Autodesk Inventor part; units mm, degrees
ref_plane "YZ Plane" through (0, 0, 0) normal (1, 0, 0) x (0, 1, 0)
ref_plane "XZ Plane" through (0, 0, 0) normal (0, 1, 0) x (-1, 0, 0)
ref_plane "XY Plane" through (0, 0, 0) normal (0, 0, 1) x (1, 0, 0)
sketch "Sketch1" plane through (0, 0, 0) normal (0, 1, 0) x (-1, 0, 0)
  circle A0 centre (0, 0) radius 57
  circle A1 centre (0, 0) radius 50
  line L0 (0, -85.4) -> (0, 113.4)
  line L1 (112.682, 0) -> (-112.682, 0)
  line L2 (-50, 2) -> (50, 2)
  line L3 (50, 2) -> (50, -2)
  line L4 (50, -2) -> (-50, -2)
  line L5 (-50, -2) -> (-50, 2)
  line L6 (-50, 2) -> (50, -2) construction
  line L7 (50, 2) -> (-50, -2) construction
  line L8 (2, 50) -> (-2, 50)
  line L9 (-2, 50) -> (-2, -50)
  line L10 (-2, -50) -> (2, -50)
  line L11 (2, -50) -> (2, 50)
  line L12 (2, 50) -> (-2, -50) construction
  line L13 (-2, 50) -> (2, -50) construction
  line L14 (13.75, 85) -> (-13.75, 85)
  line L15 (-13.75, 85) -> (-13.75, 50)
  line L16 (-13.75, 50) -> (13.75, 50)
  line L17 (13.75, 50) -> (13.75, 85)
  line L18 (0, 85) -> (0, 50) construction
  line L19 (13.75, 60) -> (-13.75, 60)
  line L20 (-44.3013, -23.2679) -> (-42.3013, -26.7321)
  line L21 (-36.4263, -36.9078) -> (-50.1763, -13.0922)
  line L22 (-58.8365, -18.0922) -> (-45.0865, -41.9078)
  line L23 (-66.7372, -54.4078) -> (-36.4263, -36.9078)
  line L24 (-50.1763, -13.0922) -> (-80.4872, -30.5922)
  line L25 (-73.6122, -42.5) -> (-43.3013, -25) construction
  line L26 (-80.4872, -30.5922) -> (-66.7372, -54.4078)
  line L27 (42.3013, -26.7321) -> (44.3013, -23.2679)
  line L28 (50.1763, -13.0922) -> (36.4263, -36.9078)
  line L29 (45.0865, -41.9078) -> (58.8365, -18.0922)
  line L30 (80.4872, -30.5922) -> (50.1763, -13.0922)
  line L31 (36.4263, -36.9078) -> (66.7372, -54.4078)
  line L32 (73.6122, -42.5) -> (43.3013, -25) construction
  line L33 (66.7372, -54.4078) -> (80.4872, -30.5922)
  point P0 (2, -49.96)
  point P1 (2, -2)
  point P2 (49.96, -2)
  point P3 (-2, 49.96)
  point P4 (-2, 2)
  point P5 (-49.96, 2)
  point P6 (-2, -49.96)
  point P7 (-49.96, -2)
  point P8 (-2, -2)
  point P9 (-13.75, 55.3167)
  point P10 (-54.7807, -15.7505)
  point P11 (-41.0307, -39.5662)
  point P12 (41.0307, -39.5662)
  point P13 (54.7807, -15.7505)
  point P14 (13.75, 55.3167)
  point P15 (2, 49.96)
  point P16 (49.96, 2)
  point P17 (2, 2)
  dimension "d0" = 114
  dimension "d1" = 100
  dimension "d6" = 100
  dimension "d7" = 4
  dimension "d8" = 4
  dimension "d9" = 100
  dimension "d10" = 27.5
  dimension "d14" = 60
  dimension "d15" = 25
  dimension "d18" = 360
extrude "Extrusion1" add sketch "Sketch1" along normal blind 5 contours L1 L3 L2 A1 L11 L16 L17 A0 | A0 L30 L28 L27 A1 L4 L3 L1 | L17 L16 L8 L0 A0 | A0 L0 L19 L17 | L30 L29 L31 A0 | A0 L31 L28 L27 L30 | L1 L11 L2 A1 | L3 L4 A1 | A1 L4 L11 L1 | A1 L2 L3 | L0 L8 L16 L15 A0 | A0 L15 L19 L0 | L19 L0 L14 L17 | A0 L0 L10 L11 A1 L27 L28 L31 | L30 L33 L31 L29 | L11 L4 L0 L1 | L1 L0 L2 L11 | L15 L16 L9 A1 L2 L5 L1 A0 | L8 L11 A1 | L0 L2 L9 A1 | A1 L11 L2 L0 | A1 L9 L8 | L19 L15 L14 L0 | A0 L23 L21 L20 A1 L9 L10 L0 | L11 A1 L0 L4 | L1 L9 L2 L0 | L0 L4 L9 L1 | L1 L5 L4 A1 L20 L21 L24 A0 | L23 L22 L24 A0 | A0 L24 L21 L20 L23 | L10 L9 A1 | A1 L9 L4 L0 | A1 L11 L10 | L9 L4 A1 L1 | L1 A1 L2 L9 | L5 L2 A1 | A1 L4 L5 | L23 L26 L24 L22
sketch "Sketch5" plane through (0, 5, 0) normal (0, 1, 0) x (1, 0, 0)
  line L0 (-2, -21.5) -> (2, -21.5)
  line L1 (2, -21.5) -> (2, -17.5)
  line L2 (2, -17.5) -> (-2, -17.5)
  line L3 (-2, -17.5) -> (-2, -21.5)
  line L4 (-2, -2) -> (-2, -49.96) construction
  line L5 (2, -49.96) -> (2, -2) construction
  line L6 (-112.682, 0) -> (112.682, 0) construction
  line L7 (-2, 21.5) -> (2, 21.5)
  line L8 (2, 21.5) -> (2, 17.5)
  line L9 (2, 17.5) -> (-2, 17.5)
  line L10 (-2, 17.5) -> (-2, 21.5)
  arc A0 (-49.96, -2) -> (-2, -49.96) centre (0, 0) ccw construction
  arc A1 (-2, 49.96) -> (-49.96, 2) centre (0, 0) ccw construction
  circle A2 centre (0, 0) radius 50 construction
  line L11 (-54, 6) -> (-50, 6)
  line L12 (-50, 6) -> (-50, -6)
  line L13 (-50, -6) -> (-54, -6)
  line L14 (-54, -6) -> (-54, 6)
  line L15 (-54, 0) -> (-50, 0) construction
  line L16 (0, 88.2024) -> (0, -113.8671) construction
  line L17 (54, 6) -> (50, 6)
  line L18 (50, 6) -> (50, -6)
  line L19 (50, -6) -> (54, -6)
  line L20 (54, -6) -> (54, 6)
  line L21 (54, 0) -> (50, 0) construction
  point P0 (49.96, -2)
  point P1 (49.96, 2)
  dimension "d41" = 17.5
  dimension "d42" = 4
  dimension "d43" = 12
extrude "Extrusion4" add sketch "Sketch5" along normal blind 10
sketch "Sketch2" plane through (0, 5, 0) normal (0, 1, 0) x (1, 0, 0)
  line L0 (-13.75, -55.3167) -> (-13.75, -85)
  line L1 (13.75, -85) -> (13.75, -55.3167)
  line L2 (-13.75, -85) -> (13.75, -85)
  line L3 (13.75, -85) -> (13.75, -61)
  line L4 (13.75, -61) -> (-13.75, -61)
  line L5 (-13.75, -61) -> (-13.75, -85)
  line L6 (-12.25, -62.5) -> (12.25, -62.5)
  line L7 (12.25, -62.5) -> (12.25, -83.5)
  line L8 (12.25, -83.5) -> (-12.25, -83.5)
  line L9 (-12.25, -83.5) -> (-12.25, -62.5)
  line L10 (80.4872, 30.5922) -> (66.7372, 54.4078)
  line L11 (66.7372, 54.4078) -> (45.9525, 42.4078)
  line L12 (45.9525, 42.4078) -> (59.7025, 18.5922)
  line L13 (59.7025, 18.5922) -> (80.4872, 30.5922)
  line L14 (60.2516, 20.6412) -> (48.0016, 41.8588)
  line L15 (48.0016, 41.8588) -> (66.1881, 52.3588)
  line L16 (66.1881, 52.3588) -> (78.4381, 31.1412)
  line L17 (78.4381, 31.1412) -> (60.2516, 20.6412)
  line L18 (-66.7372, 54.4078) -> (-80.4872, 30.5922)
  line L19 (-80.4872, 30.5922) -> (-59.7025, 18.5922)
  line L20 (-59.7025, 18.5922) -> (-45.9525, 42.4078)
  line L21 (-45.9525, 42.4078) -> (-66.7372, 54.4078)
  line L22 (-48.0016, 41.8588) -> (-60.2516, 20.6412)
  line L23 (-60.2516, 20.6412) -> (-78.4381, 31.1412)
  line L24 (-78.4381, 31.1412) -> (-66.1881, 52.3588)
  line L25 (-66.1881, 52.3588) -> (-48.0016, 41.8588)
  point P0 (0, 0)
  point P1 (-13.75, -61)
  point P2 (-13.75, -61)
  dimension "d22" = 24
  dimension "d23" = 1.5
  dimension "d26" = 360
extrude "Extrusion2" add sketch "Sketch2" along normal blind 20 contours L4 L1 L2 L0
sketch "Sketch4" plane through (-13.75, 0, 85) normal (0, 0, 1) x (1, 0, 0)
  line L0 (0, 25) -> (27.5, 25) construction
  line L1 (7.75, 25) -> (19.75, 25)
  line L2 (19.75, 25) -> (19.75, 10)
  line L3 (19.75, 10) -> (7.75, 10)
  line L4 (7.75, 10) -> (7.75, 25)
  line L5 (1.5, 5) -> (26, 5) construction
  line L6 (13.75, -10.2) -> (13.75, 61.2) construction
  circle A0 centre (13.75, 16) radius 6
  point P0 (13.75, 0)
  point P1 (7.75, 16)
  point P2 (19.75, 16)
  dimension "d36" = 12
  dimension "d37" = 5
  dimension "d38" = 6
extrude "Extrusion3" cut sketch "Sketch4" against normal up to surface (24 mm away) contours L1 L2 A0 L4 | A0
pattern_circular "Circular Pattern1" count 3 over 360 about axis through (0, -10, 0) along (0, 1, 0) of "Extrusion2", "Extrusion3"
equation "\"d38\" = 0.5 * d36"
properties part number "bottom3"
Read the model definition and answer for the solid it produces. Units are mm, in the model's axes. A direction names the side the tool comes from. Round coordinates to 2 decimals unless told otherwise and drop trailing zeros. Loops run counter-clockwise (first coordinate to the right, second up) from the corner with the lowest first, then second, coordinate; pieces in that order, holes last.
Q1. Which of the six approach directions +Z, -Z, +X, -X, +Y, -Y give full straight-line access (tool end or side, diameter ignored) to faces 4 (the face through (2, 4, -26)), 5 (the face through (-52, 10, -6)), 6 (the face through (12.25, 15, 73)), 7 (the face through (50, 10, 0)), 8 (the face through (-52, 10, 6))?
Q2. Determine the mould class of faces 1 (the face through (0, 15, -20)), 2 (the face through (52, 10, 6)), 3 (the face through (49.681, 2.465, 27.943)) for opening direction Z: released by +Z, released by -Z, zero draft, split by the parting line, or undercut.
Q3. Consider probe 1 along Z at (x, y) = (-52, 7); probe 2 along Z at (x, y) = (9, 21.5); probe 3 along Z at (x, y) = (-16, 2). Determine where each line is inside the solid, lowest interval first.
Q4. Each of these flat-tipped pins is pushed along its axis until it touches: pin 1 (0.8 mm diameter, centred on y = 21.5, z = 84.5, fed in from -X); pin 2 (2 mm diameter, centred on x = -52, y = 9, fed in from +Z); pin 3 (2.5 mm diameter, centred on x = 36.5, y = 3.5, fed in from -Z); pin 4 (10 mm diameter, centred on y = 21, z = 16, fed in from -X). Where does it stop, or does it pass through?
Q5. Section B-B on z = 44 is taken. Write down the section's boundary in (x, y), and give its area (3 significant figures).
Q6. Section A-A on y = 3 is taken. Write down the section's boundary in (x, z).
Q7. Section C-C on x = -30 is taken. Write down the section's boundary in (y, z), and give its area (3 significant figures).
Output:
1. face 4: +Y, -Y
1. face 5: +X, -X, +Y
1. face 6: +Y
1. face 7: +Z, +Y
1. face 8: +Z, +X, -X, +Y
2. face 1: zero draft
2. face 2: released by +Z
2. face 3: undercut
3. probe 1: z = -45.9 to -44.17, -34.93 to -31.93, -6 to 6
3. probe 2: z = 61 to 62.5, 83.5 to 85
3. probe 3: z = -54.71 to -47.37, -2 to 2, 47.37 to 54.71
4. pin 1: stops at x = -13.75
4. pin 2: stops at z = 6
4. pin 3: stops at z = -44.79
4. pin 4: passes through
5. outline: (-36.24, 0) - (-23.75, 0) - (-23.75, 5) - (-36.24, 5) - close; (-2, 0) - (2, 0) - (2, 5) - (-2, 5) - close; (23.75, 0) - (36.24, 0) - (36.24, 5) - (23.75, 5) - close
5. area: 145 mm2
6. outline: (-80.49, -30.59) - (-66.74, -54.41) - (-41.03, -39.57) arc R57 ccw to (41.03, -39.57) - (66.74, -54.41) - (80.49, -30.59) - (54.78, -15.75) arc R57 ccw to (13.75, 55.32) - (13.75, 85) - (-13.75, 85) - (-13.75, 55.32) arc R57 ccw to (-54.78, -15.75) - close; hole (-49.96, -2) arc R50 ccw to (-2, -49.96) - (-2, -2) - close; hole (-49.96, 2) - (-2, 2) - (-2, 49.96) arc R50 ccw to start; hole (2, -49.96) arc R50 ccw to (49.96, -2) - (2, -2) - close; hole (2, 2) - (49.96, 2) arc R50 ccw to (2, 49.96) - close
7. outline: (0, -48.47) - (5, -48.47) - (5, -40) - (0, -40) - close; (0, -2) - (5, -2) - (5, 2) - (0, 2) - close; (0, 40) - (5, 40) - (5, 48.47) - (0, 48.47) - close
7. area: 105 mm2
